from build123d import *

# Parameters (mm, degrees)
F1_DEPTH = 50
F2_W     = 55
F2_H     = 77
F3_DEPTH = 100
F5_DEPTH = 90


with BuildPart() as f1:
    # F0 (on Top) → F1 (new body)
    with BuildSketch(Plane.XY):
        Polygon((-36.420125, 59.16098), (-46.420125, 59.16098), (-46.420125, -32.83902), (93.579875, -32.83902), (93.579875, 59.16098), (83.579875, 59.16098), (83.579875, -17.83902), (28.579875, -17.83902), (28.579875, 59.16098), (18.579875, 59.16098), (18.579875, -17.83902), (-36.420125, -17.83902), align=None)
    extrude(amount=F1_DEPTH)

    # F2 (on face) → F3 (join)
    with BuildSketch(Plane.XY.offset(50)):
        with Locations((-8.920125, 20.66098)):
            Rectangle(F2_W, F2_H)
        Polygon((-36.420125, -17.83902), (-36.420125, 59.16098), (-46.420125, 59.16098), (-46.420125, -32.83902), (93.579875, -32.83902), (93.579875, 59.16098), (83.579875, 59.16098), (83.579875, -17.83902), (28.579875, -17.83902), (28.579875, 59.16098), (18.579875, 59.16098), (18.579875, -17.83902), align=None)
    extrude(amount=F3_DEPTH)

    # F4 (on face) → F5 (cut)
    with BuildSketch(Plane.XY.offset(150)):
        Polygon((28.579875, 59.16098), (-36.420125, 59.16098), (-36.420125, -17.760558), (8.856312, -17.760558), (28.579875, -17.83902), align=None)
    extrude(amount=-F5_DEPTH, mode=Mode.SUBTRACT)


solid = f1.part
Check sheet for the modelled part. Datum: model origin and axes. Units: mm. A direction names the side the tool comes from. Round coordinates to 2 decimals unless told otherwise and drop trailing zeros. Order: outer loops, then holes, each group sorted by start corner. A loop starts at its lowest first (then second) coordinate and runs counter-clockwise, first axis right, second up.
(1) Cross-section at C-C, the plane x = -7.5. Enter the section's corners in (y, z).
(2) Draft check along X on faces 1 (the flat face through (-9, 21, 50)), 2 (the flat face through (93.58, 13, 74)), 3 (the flat face through (23, 4, 0)), 4 (the flat face through (-36.42, 21, 106)). Enter one of: pulls with the +X half, pulls with the -X half, needs draft (parallel to the pull), parting line crosses it, or undercut.
(3) Cross-section at B-B, the plane z = 79. Enter the section's corners in (x, y).
(4) Go/stop test with flat-tipped pins: P1, Ø10, axis at x = -9, z = 106, coming from the +Y side; P2, Ø6, axis at x = 5, y = 20.5, coming from the -Z side; P3, Ø3, axis at x = 20, y = 36.5, coming from the +Z side. Record where each tip stops, or that it passes through.
(5) Cross-section at D-D, the plane z = 45.5. Enter the section's corners in (x, y), and give its area (3 significant figures).
(6) Cross-section at A-A, the plane y = 48.5. Enter the section's corners in (x, z).
(7) Scan lines: probe 1 along X at (y, z) = (17, 12); probe 2 along X at (y, z) = (-9, 59.5); probe 3 along X at (y, z) = (-9, 144). Record each from-to range of solid material in increasing order.
(8) Access from +Z, -Z, +X, -X, +Y, -Y to the whole of each face (thin tool, end or side, straight path). Record for faces 5 (the flat face through (28, -21, 150)), 6 (the flat face through (-20, 59.161, 58)), 7 (the flat face through (-9, -17.839, 25)), 8 (the flat face through (56, -17.839, 74)), 9 (the flat face through (-14, -17.761, 106)).
Check sheet entries:
1. outline: (-32.84, 0) - (-17.84, 0) - (-17.84, 50) - (59.16, 50) - (59.16, 60) - (-17.76, 60) - (-17.76, 150) - (-32.84, 150) - close
2. face 1: undercut
2. face 2: pulls with the +X half
2. face 3: needs draft
2. face 4: undercut
3. outline: (-46.42, -32.84) - (93.58, -32.84) - (93.58, 59.16) - (83.58, 59.16) - (83.58, -17.84) - (28.58, -17.84) - (8.86, -17.76) - (-36.42, -17.76) - (-36.42, 59.16) - (-46.42, 59.16) - close
4. P1: stops at y = -17.76
4. P2: stops at z = 50
4. P3: stops at z = 60
5. outline: (-46.42, -32.84) - (93.58, -32.84) - (93.58, 59.16) - (83.58, 59.16) - (83.58, -17.84) - (28.58, -17.84) - (28.58, 59.16) - (18.58, 59.16) - (18.58, -17.84) - (-36.42, -17.84) - (-36.42, 59.16) - (-46.42, 59.16) - close
5. area: 4,410 mm2
6. outline: (-46.42, 0) - (-36.42, 0) - (-36.42, 50) - (18.58, 50) - (18.58, 0) - (28.58, 0) - (28.58, 60) - (-36.42, 60) - (-36.42, 150) - (-46.42, 150) - close; (83.58, 0) - (93.58, 0) - (93.58, 150) - (83.58, 150) - close
7. probe 1: x = -46.42 to -36.42, 18.58 to 28.58, 83.58 to 93.58
7. probe 2: x = -46.42 to 28.58, 83.58 to 93.58
7. probe 3: x = -46.42 to -36.42, 83.58 to 93.58
8. face 5: +Z, +X, -X, +Y, -Y
8. face 6: +Z, -Z, +X, -X, +Y
8. face 7: -Z, +Y
8. face 8: +Z, -Z, +Y
8. face 9: +Z, +Y
